CAD build for the part. Positions are in the model's coordinates, mm. Give positions to 0.01 mm unless a question says otherwise; leave off trailing zeros. Order: outer loops, then holes, each group sorted by start corner. A loop starts at its lowest first (then second) coordinate and runs counter-clockwise, first axis right, second up. Notation, with made-up numbers: (77.5, -14) -> (105.5, -14) arc R13 ccw to (105.5, -9) -> close; hole circle Ø7 at (54.5, 22). An arc over 180 degrees is marked (long way). Use one line per item in the form item = value. Start each with the question number.
1) Probe line 1 (X direction, y = 0, z = 2); line 2 (X direction, y = -4.25, z = -4.25); line 3 (Y direction, x = 4.5, z = 2). List the from-to ranges inside material, lowest first.
2) Drop flat-ended pins along their axis: P1, Ø1.5, axis at y = -7.5, z = -5, coming from the -X side; P2, Ø1.5, axis at y = -8.5, z = 2.5, coming from the +X side. Give the stop position or say it passes through.
3) Cut at B-B, the plane y = 5. Give the cut face in (x, z), and give its area (3 significant figures).
4) Cut at A-A, the plane z = 2.75. Give the cut face in (x, y).
Autodesk Inventor part; units mm, degrees
ref_plane "Work Plane1" through (0, 0, -9) normal (0, 0, 1) x (1, 0, 0)
ref_plane "Work Plane2" through (0, 0, 5) normal (0, 0, 1) x (1, 0, 0)
ref_plane "Work Plane3" through (90, 0, 5) normal (1, 0, 0) x (0, 1, 0)
sketch "Sketch1" plane through (0, 0, 0) normal (0, 0, 1) x (1, 0, 0)
  line L0 (11, 11) -> (79, 11)
  line L1 (79, -11) -> (11, -11)
  arc A0 (11, 11) -> (11, -11) centre (11, 0) ccw
  line L2 (0, 9.4) -> (0, -7.4)
  line L3 (-5, 0) -> (30, 0)
  arc A1 (79, -11) -> (79, 11) centre (79, 0) ccw
  line L4 (90, 0) -> (90, 7) construction
  dimension "d0" = 11
  dimension "d8" = 11
  dimension "d9" = 90
ref_plane "Work Plane1" through (0, 0, -9) normal (0, 0, 1) x (1, 0, 0)
ref_plane "Work Plane2" through (0, 0, 5) normal (0, 0, 1) x (1, 0, 0)
extrude "Body1" add sketch "Sketch1" against normal up to surface (14 mm away) from surface at 5
ref_plane "Work Plane3" through (90, 0, 5) normal (1, 0, 0) x (0, 1, 0)
equation "\"d0\" = 0.5 * PB"
equation "\"d8\" = 0.5 * PB"
equation "\"d9\" = NLG"
equation "\"d1\" = -PNT"
equation "\"d2\" = PH - PNT"
equation "\"NLG\" = 90"
equation "\"PB\" = 22"
equation "\"PNT\" = 9"
equation "\"PH\" = 14"
equation "\"RR\" = 0.001"
equation "\"WDMIN\" = 75"
equation "\"PHH\" = 0"
equation "\"WDMAX\" = 85"
equation "\"PUEB\" = 5.4"
properties part number "DIN 6885 - A 22 x 14 x 90" material "Steel, Mild"
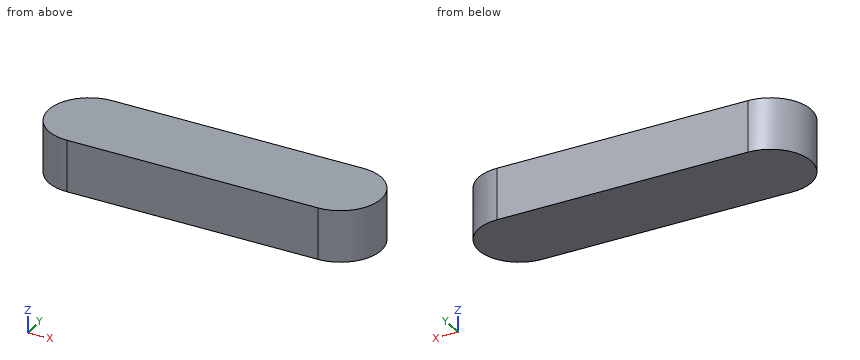
Result:
q1.line_1 = 0 to 90
q1.line_2 = 0.85 to 89.15
q1.line_3 = -8.87 to 8.87
q2.P1 = 2.31
q2.P2 = 86.81
q3.outline = (1.2, -9) -> (88.8, -9) -> (88.8, 5) -> (1.2, 5) -> close
q3.area = 1,230 mm²
q4.outline = (11, -11) -> (79, -11) arc R11 ccw to (79, 11) -> (11, 11) arc R11 ccw to start
